Work out the finished part from the listing and answer in its coordinate system (mm). A direction names the side the tool comes from. Coordinates: 2 decimals unless noted, no trailing zeros. Order: outer loops, then holes, each group sorted by start corner. A loop starts at its lowest first (then second) coordinate and runs counter-clockwise, first axis right, second up. Notation, with made-up numbers: M -5.5,19 L 42.5,19 A17 ccw 42.5,24 Z; hole C 52,41.5 d4. An arc over 180 degrees is marked long. Answer in a Markdown table with one row per item. Add a question column.
Item 1: Which of the six approach directions +Z, -Z, +X, -X, +Y, -Y give full straight-line access (tool end or side, diameter ignored) to faces 1 (the face through (-23, -16, 38.1)), 2 (the face through (18.14, 7.42, 0))?
Item 2: Flat-ended cylindrical pins translate along their axes: pin 1 Ø6 at (y, z) = (10.5, 17.5) entering from -X; pin 2 Ø6 at (x, z) = (5.5, 20) entering from +Y; pin 3 Ø18 at (x, y) = (9, 5) entering from -Z. Find the tip coordinate at first contact, or state that the pin passes through.
Item 3: Consider line 1 (Y direction, x = 0, z = 11); line 2 (Z direction, x = 0, y = 24); line 3 (Y direction, x = 14.5, z = 15). Determine where each line is inside the solid, lowest interval first. Write a range as from..to.
Item 4: The part is cut by section A-A (x = 0). State how many separate pieces and enclosed holes the cut face has, then the cut area to 3 significant figures.
Item 5: The mould has two halves that part along Y. Classify faces 3 (the face through (-3.66, -16.49, 21.32)), 4 (the face through (-5.892, -26.532, 20.071)), 5 (the face through (-5.037, 21.572, 16.732)): released by +Y, released by -Y, zero draft, split by the parting line, or undercut.
Item 6: The part is cut by section D-D (z = 16.51). Write down the section's boundary in (x, y), then the cut area to 3 significant figures.
Item 7: The part is cut by section C-C (z = 25). Write down the section's boundary in (x, y).
from build123d import *

# Parameters (mm, degrees)
F0_R     = 27.178
F0_R_2   = 16.891
F1_DEPTH = 38.1
F2_R     = 30.353
F2_R_2   = 27.178
F2_R_3   = 16.891
F3_DEPTH = 5.08
F5_D     = 10.0838
F5_DEPTH = 30.354
F6_R     = 2.54
F7_R     = 5.07999


# Not quite as in the source:
# - a fillet or chamfer is up to 0.001 mm smaller than in the source, because OpenCascade refuses the exact size


with BuildPart() as f1:
    # F0 (on Top) → F1 (new body)
    with BuildSketch(Plane.XY):
        Circle(F0_R)
        Circle(F0_R_2, mode=Mode.SUBTRACT)
    extrude(amount=F1_DEPTH)

    # F2 (on face) → F3 (join)
    with BuildSketch(Plane.XY.offset(38.1)):
        Circle(F2_R)
        Circle(F2_R_2, mode=Mode.SUBTRACT)
        Circle(F2_R_2)
        Circle(F2_R_3, mode=Mode.SUBTRACT)
    extrude(amount=F3_DEPTH)

    # F5 (through all, one way)
    with BuildSketch(Plane.XZ):
        with Locations((0, 16.51)):
            Circle(F5_D / 2)
    extrude(amount=-F5_DEPTH, mode=Mode.SUBTRACT)

    # F6
    f6_edges = [f1.edges().sort_by_distance(p)[0] for p in [
        (-16.891, 0, 0),
        (-27.178, 0, 0),
        (-16.891, 0, 43.18),
    ]]
    fillet(f6_edges, radius=F6_R)

    # F7 (radius 5.08 in the source; OpenCascade refuses exactly that, so slightly less here)
    f7_edges = [f1.edges().sort_by_distance(p)[0] for p in [
        (-30.353, 0, 43.18),
    ]]
    fillet(f7_edges, radius=F7_R)


solid = f1.part
Reply:
| question | item | result |
|---|---|---|
| 1 | face 1 | -Z |
| 1 | face 2 | -Z, +X, -X, +Y, -Y |
| 2 | pin 1 | stops at x = -26.12 |
| 2 | pin 2 | stops at y = 27.05 |
| 2 | pin 3 | stops at z = 0 |
| 3 | line 1 | y = -27.18..-16.89, 16.89..27.18 |
| 3 | line 2 | z = 0..11.47, 21.55..43.18 |
| 3 | line 3 | y = -22.99..-8.66, 8.66..22.99 |
| 4 | separate pieces | 3 |
| 4 | enclosed holes | 0 |
| 4 | area | 798 mm2 |
| 5 | face 3 | undercut |
| 5 | face 4 | split by the parting line |
| 5 | face 5 | zero draft |
| 6 | outline | M -5.04,16.12 L -5.04,26.71 A27.18 ccw long 5.04,26.71 L 5.04,16.12 A16.89 cw long Z |
| 6 | area | 1,320 mm2 |
| 7 | outline | C 0,0 d54.36; hole C 0,0 d33.78 |
